Could you check a few things on this model? Use its own coordinates, in mm. A direction names the side the tool comes from. Coordinates: 2 decimals unless noted, no trailing zeros. Loops run counter-clockwise (first coordinate to the right, second up) from the corner with the lowest first, then second, coordinate; pieces in that order, holes last. Notation, with made-up numbers: (49.25, 88) -> (70.25, 88) arc R17 ccw to (70.25, 110) -> close; hole circle Ø1 at (1, 49.5). An arc over 180 degrees is marked (long way). One line per question, with ' | ' between items.
Autodesk Inventor part; units mm, degrees
ref_plane "YZ Plane" through (0, 0, 0) normal (1, 0, 0) x (0, 1, 0)
ref_plane "XZ Plane" through (0, 0, 0) normal (0, 1, 0) x (-1, 0, 0)
ref_plane "XY Plane" through (0, 0, 0) normal (0, 0, 1) x (1, 0, 0)
sketch "Esquisse1" plane through (0, 0, 0) normal (0, 0, 1) x (1, 0, 0)
  line L0 (0, 8) -> (0, 5)
  arc A0 (24.3671, 0.2221) -> (0, 5) centre (0, -59.525) ccw
  arc A1 (24.3671, 0.2221) -> (28.5, 3) centre (25.5, 3) ccw
  line L1 (28.5, 3) -> (28.5, 189.1581)
  arc A2 (28.5, 189.1581) -> (27.143, 192.5828) centre (23.5, 189.1581) ccw
  line L2 (27.143, 192.5828) -> (15, 205.5)
  line L3 (15, 205.5) -> (15, 227)
  line L4 (15, 227) -> (10.75, 227)
  line L5 (10.75, 227) -> (10.75, 207.6222)
  arc A3 (10.75, 207.6222) -> (12.107, 204.1975) centre (15.75, 207.6222) ccw
  line L6 (12.107, 204.1975) -> (24.143, 191.3941)
  arc A4 (25.5, 187.9694) -> (24.143, 191.3941) centre (20.5, 187.9694) ccw
  line L7 (25.5, 187.9694) -> (25.5, 10)
  arc A5 (23.5, 8) -> (25.5, 10) centre (23.5, 10) ccw
  line L8 (23.5, 8) -> (0, 8)
  line L9 (0, 0) -> (25.5, 0) construction
  point P0 (28.1484, 191)
  dimension "d0" = 57
  dimension "d1" = 30
  dimension "d2" = 21.5
  dimension "d3" = 21.5
  dimension "d4" = 3
  dimension "d5" = 3
  dimension "d6" = 14.5
  dimension "d7" = 5
  dimension "d8" = 3
  dimension "d9" = 3
  dimension "d10" = 2
  dimension "d11" = 227
  dimension "d12" = 5
revolve "Révolution1" add sketch "Esquisse1" angle 360 about axis through (0, 8, 0) along (0, -1, 0)
equation "\"d5\" = d4"
properties part number "Bouteille" material "Verre"
Q1. For pin 1 (1 mm diameter, centred on x = -21, z = -4, fed in from -Y); pin 2 (1 mm diameter, centred on x = 0, y = 54, fed in from -Z); pin 3 (1.5 mm diameter, centred on y = 156, z = 6.5, fed in from -X), each with a flat end and sliding along its axis, tell me the tip position at first contact or that it passes through.
Values follow:
pin 1: stops at y = 1.18 | pin 2: stops at z = -28.5 | pin 3: stops at x = -27.91
Q2. For faces 4 (the face through (10, 227, -6)), 5 (the face through (-2.79, 203.4, -12.55)), 6 (the face through (-14.985, 216.4, -0.66)), which set-ups out of +Z, -Z, +X, -X, +Y, -Y let a thin tool reach every point of the face, with its end or its side?
Values follow:
face 4: +Z, -Z, +X, -X, +Y | face 5: none | face 6: +Y
Q3. We'd pull the mould along Y, two halves only. Please class faces 1 (the face through (0, 8, 0)), 2 (the face through (-1.4, 217.18, 10.66)), 3 (the face through (15.032, 204.692, 4.734)): released by +Y, released by -Y, zero draft, split by the parting line, or undercut.
Values follow:
face 1: undercut | face 2: zero draft | face 3: released by +Y
Q4. Imagine slicing it at A-A on y = 43. Write out the boundary of the cut face in (x, z).
Values follow:
outline: circle Ø57 at (0, 0); hole circle Ø51 at (0, 0)
Q5. Please list where these lines run through material, in increasing order: L1, parallel to Z at x = 0, y = 51; L2, parallel to Z at x = 0, y = 214; L3, parallel to X at y = 48, z = 6.5. Write a range as [from, to].
Values follow:
L1: z = [-28.5, -25.5], [25.5, 28.5] | L2: z = [-15, -10.75], [10.75, 15] | L3: x = [-27.75, -24.66], [24.66, 27.75]
